Source: CAD feature listing. Evaluate the final solid. Frame: model axes, mm. Face numbers are marked on the shaded views. A direction names the side the tool comes from. Coordinates: 2 decimals unless noted, no trailing zeros. Loops run counter-clockwise (first coordinate to the right, second up) from the corner with the lowest first, then second, coordinate; pieces in that order, holes last. Notation, with made-up numbers: (82, -30.5) -> (97, -30.5) arc R7 cw to (97, -17.5) -> close; hole circle Ø7 at (56, 19). An arc over 180 degrees is marked (long way). Answer as CSV lines item,"result".
from build123d import *

# Parameters (mm, degrees)
SM_BASE_FLANGE_1_DEPTH = 70
SKETCH_3_R             = 31
SKETCH_3_R_2           = 3.25
CUT_EXTRUDE_1_DEPTH    = 2
SKETCH_4_W             = 149
SKETCH_4_H             = 2
EXTRUDE_2_DEPTH        = 15
SKETCH_5_W             = 149
SKETCH_5_H             = 2
EXTRUDE_3_DEPTH        = 15


# Sheet-metal steps are written as plain solids
with BuildPart() as part:
    # Sketch 1 → Базовая кромка1 (new, symmetric)
    with BuildSketch(Plane.XY):
        with BuildLine():
            Line((0, 0), (175, 0))
            ThreePointArc((175, 0), (177.828427125, -1.171572875), (179, -4))
            Line((179, -4), (179, -20))
            Line((179, -20), (177, -20))
            Line((177, -20), (177, -4))
            ThreePointArc((177, -4), (176.414213562, -2.585786438), (175, -2))
            Line((175, -2), (0, -2))
            Line((0, -2), (0, 0))
        make_face()
    extrude(amount=SM_BASE_FLANGE_1_DEPTH, both=True)

    # Эскиз3 → Вытянуть1 (cut)
    with BuildSketch(Plane(origin=(0, 0, 0), x_dir=(1, 0, 0), z_dir=(0, 1, 0))):
        with Locations(Location((59.5, 0, 0), (0, 0, 270))):
            Circle(SKETCH_3_R)
        with Locations(Location((6, 50, 0), (0, 0, 270))):
            Circle(SKETCH_3_R_2)
        with Locations(Location((6, 0, 0), (0, 0, 270))):
            Circle(SKETCH_3_R_2)
        with Locations(Location((6, -50, 0), (0, 0, 270))):
            Circle(SKETCH_3_R_2)
    extrude(amount=-CUT_EXTRUDE_1_DEPTH, mode=Mode.SUBTRACT)

    # Эскиз4 → Вытянуть2 (add)
    with BuildSketch(Plane.XY.offset(70)):
        with Locations((89.5, -1)):
            Rectangle(SKETCH_4_W, SKETCH_4_H)
    extrude(amount=EXTRUDE_2_DEPTH)

    # Эскиз5 → Вытянуть3 (add)
    with BuildSketch(Plane(origin=(0, 0, -70), x_dir=(-1, 0, 0), z_dir=(0, 0, -1))):
        with Locations((-89.5, -1)):
            Rectangle(SKETCH_5_W, SKETCH_5_H)
    extrude(amount=EXTRUDE_3_DEPTH)

    # Эскиз8 → Зенковка для винта с потайной головкой M61 (revolve, cut)
    with BuildSketch(Plane(origin=(34.5, 0, 77.5), x_dir=(0, 0, 1), z_dir=(1, 0, 0))):
        Polygon((0, 0), (0, 2), (4.5, 2), (4.5, 1.5), (6, 0), align=None)
    revolve(axis=Axis((34.5, 6.35, 77.5), (0, -1, 0)), mode=Mode.SUBTRACT)

    # Эскиз8 at point 2 (carried to point 2, square into its face) → Зенковка для винта с потайной головкой M61 at 2 (revolve, cut)
    with BuildSketch(Plane(origin=(89.5, 0, 77.5), x_dir=(0, 0, 1), z_dir=(1, 0, 0))):
        Polygon((0, 0), (0, 2), (4.5, 2), (4.5, 1.5), (6, 0), align=None)
    revolve(axis=Axis((89.5, 6.35, 77.5), (0, -1, 0)), mode=Mode.SUBTRACT)

    # Эскиз8 at point 3 (carried to point 3, square into its face) → Зенковка для винта с потайной головкой M61 at 3 (revolve, cut)
    with BuildSketch(Plane(origin=(144.5, 0, 77.5), x_dir=(0, 0, 1), z_dir=(1, 0, 0))):
        Polygon((0, 0), (0, 2), (4.5, 2), (4.5, 1.5), (6, 0), align=None)
    revolve(axis=Axis((144.5, 6.35, 77.5), (0, -1, 0)), mode=Mode.SUBTRACT)

    # Эскиз8 at point 4 (carried to point 4, square into its face) → Зенковка для винта с потайной головкой M61 at 4 (revolve, cut)
    with BuildSketch(Plane(origin=(31.922835534, 0, 27.577164466), x_dir=(0, 0, 1), z_dir=(1, 0, 0))):
        Polygon((0, 0), (0, 2), (4.5, 2), (4.5, 1.5), (6, 0), align=None)
    revolve(axis=Axis((31.922835534, 6.35, 27.577164466), (0, -1, 0)), mode=Mode.SUBTRACT)

    # Эскиз8 at point 5 (carried to point 5, square into its face) → Зенковка для винта с потайной головкой M61 at 5 (revolve, cut)
    with BuildSketch(Plane(origin=(87.077164466, 0, 27.577164466), x_dir=(0, 0, 1), z_dir=(1, 0, 0))):
        Polygon((0, 0), (0, 2), (4.5, 2), (4.5, 1.5), (6, 0), align=None)
    revolve(axis=Axis((87.077164466, 6.35, 27.577164466), (0, -1, 0)), mode=Mode.SUBTRACT)

    # Эскиз8 at point 6 (carried to point 6, square into its face) → Зенковка для винта с потайной головкой M61 at 6 (revolve, cut)
    with BuildSketch(Plane(origin=(87.077164466, 0, -27.577164466), x_dir=(0, 0, 1), z_dir=(1, 0, 0))):
        Polygon((0, 0), (0, 2), (4.5, 2), (4.5, 1.5), (6, 0), align=None)
    revolve(axis=Axis((87.077164466, 6.35, -27.577164466), (0, -1, 0)), mode=Mode.SUBTRACT)

    # Эскиз8 at point 7 (carried to point 7, square into its face) → Зенковка для винта с потайной головкой M61 at 7 (revolve, cut)
    with BuildSketch(Plane(origin=(31.922835534, 0, -27.577164466), x_dir=(0, 0, 1), z_dir=(1, 0, 0))):
        Polygon((0, 0), (0, 2), (4.5, 2), (4.5, 1.5), (6, 0), align=None)
    revolve(axis=Axis((31.922835534, 6.35, -27.577164466), (0, -1, 0)), mode=Mode.SUBTRACT)

    # Эскиз8 at point 8 (carried to point 8, square into its face) → Зенковка для винта с потайной головкой M61 at 8 (revolve, cut)
    with BuildSketch(Plane(origin=(34.5, 0, -77.5), x_dir=(0, 0, 1), z_dir=(1, 0, 0))):
        Polygon((0, 0), (0, 2), (4.5, 2), (4.5, 1.5), (6, 0), align=None)
    revolve(axis=Axis((34.5, 6.35, -77.5), (0, -1, 0)), mode=Mode.SUBTRACT)

    # Эскиз8 at point 9 (carried to point 9, square into its face) → Зенковка для винта с потайной головкой M61 at 9 (revolve, cut)
    with BuildSketch(Plane(origin=(89.5, 0, -77.5), x_dir=(0, 0, 1), z_dir=(1, 0, 0))):
        Polygon((0, 0), (0, 2), (4.5, 2), (4.5, 1.5), (6, 0), align=None)
    revolve(axis=Axis((89.5, 6.35, -77.5), (0, -1, 0)), mode=Mode.SUBTRACT)

    # Эскиз8 at point 10 (carried to point 10, square into its face) → Зенковка для винта с потайной головкой M61 at 10 (revolve, cut)
    with BuildSketch(Plane(origin=(144.5, 0, -77.5), x_dir=(0, 0, 1), z_dir=(1, 0, 0))):
        Polygon((0, 0), (0, 2), (4.5, 2), (4.5, 1.5), (6, 0), align=None)
    revolve(axis=Axis((144.5, 6.35, -77.5), (0, -1, 0)), mode=Mode.SUBTRACT)

    # Эскиз8 at point 11 (carried to point 11, square into its face) → Зенковка для винта с потайной головкой M61 at 11 (revolve, cut)
    with BuildSketch(Plane(origin=(179, -12, 50), x_dir=(0, 0, 1), z_dir=(0, -1, 0))):
        Polygon((0, 0), (0, 2), (4.5, 2), (4.5, 1.5), (6, 0), align=None)
    revolve(axis=Axis((185.35, -12, 50), (-1, 0, 0)), mode=Mode.SUBTRACT)

    # Эскиз8 at point 12 (carried to point 12, square into its face) → Зенковка для винта с потайной головкой M61 at 12 (revolve, cut)
    with BuildSketch(Plane(origin=(179, -12, 0), x_dir=(0, 0, 1), z_dir=(0, -1, 0))):
        Polygon((0, 0), (0, 2), (4.5, 2), (4.5, 1.5), (6, 0), align=None)
    revolve(axis=Axis((185.35, -12, 0), (-1, 0, 0)), mode=Mode.SUBTRACT)

    # Эскиз8 at point 13 (carried to point 13, square into its face) → Зенковка для винта с потайной головкой M61 at 13 (revolve, cut)
    with BuildSketch(Plane(origin=(179, -12, -50), x_dir=(0, 0, 1), z_dir=(0, -1, 0))):
        Polygon((0, 0), (0, 2), (4.5, 2), (4.5, 1.5), (6, 0), align=None)
    revolve(axis=Axis((185.35, -12, -50), (-1, 0, 0)), mode=Mode.SUBTRACT)


solid = part.part
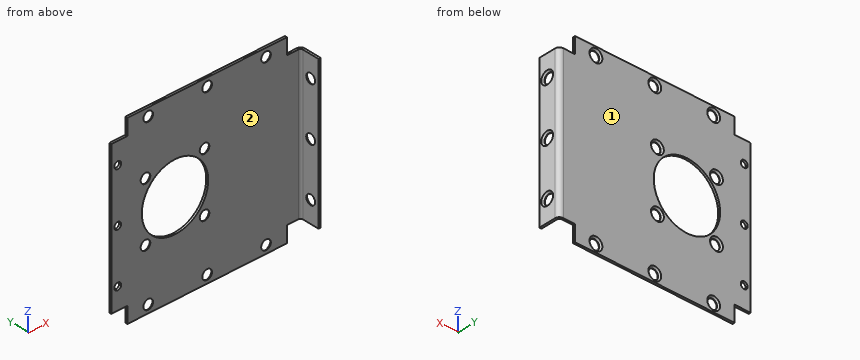
(1) Material intervals for L1, parallel to Z at x = 144.5, y = -1.8; L2, parallel to X at y = -1.55, z = 77.5; L3, parallel to X at y = -10, z = -21, sorted ascending. Write a range as [from, to].
Computed values:
L1,"[-85, -82], [-73, 73], [82, 85]"
L2,"[15, 30], [39, 85], [94, 140], [149, 164]"
L3,"[177, 179]"
(2) Cut plane A-A (x = 144.5). Return the cut outline in (y, z), then the cut area to 4 significant figures.
Computed values:
outline,"(-2, -85) -> (0, -85) -> (0, -83.5) -> (-1.5, -82) -> (-2, -82) -> close; (-2, -73) -> (-1.5, -73) -> (0, -71.5) -> (0, 71.5) -> (-1.5, 73) -> (-2, 73) -> close; (-2, 82) -> (-1.5, 82) -> (0, 83.5) -> (0, 85) -> (-2, 85) -> close"
area,"299.5 mm^2"
(3) Cut plane D-D (x = 59.5). Return the cut outline in (y, z), then the cut area to 3 significant figures.
Computed values:
outline,"(-2, -85) -> (0, -85) -> (0, -31) -> (-2, -31) -> close; (-2, 31) -> (0, 31) -> (0, 85) -> (-2, 85) -> close"
area,"216 mm^2"
(4) Cut plane C-C (z = 50). Return the cut outline in (x, y), then the cut area to 3 significant figures.
Computed values:
outline,"(0, -2) -> (2.75, -2) -> (2.75, 0) -> (0, 0) -> close; (9.25, -2) -> (175, -2) arc R2 cw to (177, -4) -> (177, -7.5) -> (177.5, -7.5) -> (179, -6) -> (179, -4) arc R4 ccw to (175, 0) -> (9.25, 0) -> close; (177, -20) -> (179, -20) -> (179, -18) -> (177.5, -16.5) -> (177, -16.5) -> close"
area,"358 mm^2"
(5) Access query for the marked faces 1 and 2. Directions: +Z, -Z, +X, -X, +Y, -Y. A direction counts if a zero-diameter tool reaches every point of the face in a straight line with its end or side. Return the directions, or none.
Computed values:
face 1,"+Z, -Z, +X, -X, +Y"
face 2,"+Z, -Z, -X, -Y"
(6) Pin query (flat end, axial travel): pin 1 Ø1 at (y, z) = (-1, 80.5) entering from -X; pin 2 Ø2 at (x, z) = (113, 27.5) entering from -Y; pin 3 Ø5 at (y, z) = (-11.5, -11.5) entering from -X; pin 4 Ø14.5 at (x, z) = (34.5, 77.5) entering from +Y. Return the tip coordinate at first contact, or that it passes through.
Computed values:
pin 1,"x = 15"
pin 2,"y = -2"
pin 3,"x = 177"
pin 4,"y = 0"
(7) Cut plane B-B (z = -77.5). Return the cut outline in (x, y), then the cut area to 3 significant figures.
Computed values:
outline,"(15, -2) -> (30, -2) -> (30, -1.5) -> (28.5, 0) -> (15, 0) -> close; (39, -2) -> (85, -2) -> (85, -1.5) -> (83.5, 0) -> (40.5, 0) -> (39, -1.5) -> close; (94, -2) -> (140, -2) -> (140, -1.5) -> (138.5, 0) -> (95.5, 0) -> (94, -1.5) -> close; (149, -2) -> (164, -2) -> (164, 0) -> (150.5, 0) -> (149, -1.5) -> close"
area,"237 mm^2"
